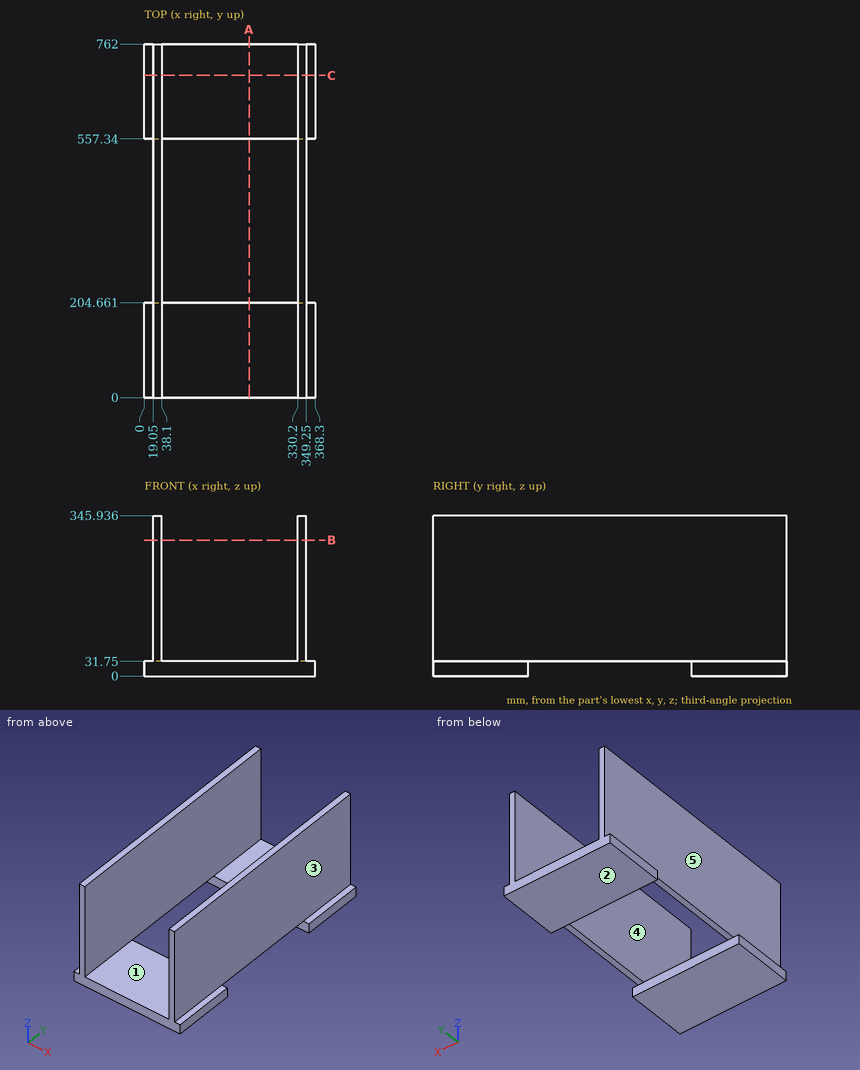
The drawing under review shows one solid part. Ordinate dimensions are in mm from its lowest x, y, z. A direction names the side the tool comes from. Coordinates: 2 decimals unless noted, no trailing zeros. Order: outer loops, then holes, each group sorted by start corner. A loop starts at its lowest first (then second) coordinate and runs counter-clockwise, first axis right, second up. Notation, with made-up numbers: (-21, 60) -> (23, 60) arc R16 ccw to (23, 88) -> close; hole circle Ø2 at (-19.5, 63.5). An arc over 180 degrees is marked (long way). One line per item, written item: value.
1) We need section B-B, the plane z = 293. Give the boundary of the cut face in (x, y), then the cut area to 3 significant figures.
Output values:
outline: (19.05, 0) -> (38.1, 0) -> (38.1, 762) -> (19.05, 762) -> close; (330.2, 0) -> (349.25, 0) -> (349.25, 762) -> (330.2, 762) -> close
area: 29,000 mm2
2) To check wall thickness, follow probe 1 along X at (y, z) = (91, 131); probe 2 along Z at (x, y) = (287.5, 100); probe 3 along Y at (x, z) = (144.5, 22.5). State the ranges of each line that lie inside material, in increasing order. Write a range as [from, to].
Output values:
probe 1: x = [19.05, 38.1], [330.2, 349.25]
probe 2: z = [0, 31.75]
probe 3: y = [0, 204.66], [557.34, 762]
3) Machinability: for the marked faces 1 and 2, which of the approach directions +Z, -Z, +X, -X, +Y, -Y give a long, thin tool a straight path to every point of the face, cutting with its end or side? Answer none if there is none.
Output values:
face 1: +Z, +Y, -Y
face 2: -Z, +X, -X, +Y, -Y
4) Draft analysis for pull direction X (two halves, no side actions). For the marked faces 3, 4 and 5, state which applies: +X half, -X half, draft (parallel to the pull), parting line (faces both ways), or undercut.
Output values:
face 3: +X half
face 4: undercut
face 5: -X half
5) We need section A-A, the plane x = 226. Give the boundary of the cut face in (y, z).
Output values:
outline: (0, 0) -> (204.66, 0) -> (204.66, 31.75) -> (0, 31.75) -> close; (557.34, 0) -> (762, 0) -> (762, 31.75) -> (557.34, 31.75) -> close
6) We need section C-C, the plane y = 694.5. Give the boundary of the cut face in (x, z), then the cut area to 3 significant figures.
Output values:
outline: (0, 0) -> (368.3, 0) -> (368.3, 31.75) -> (349.25, 31.75) -> (349.25, 345.94) -> (330.2, 345.94) -> (330.2, 31.75) -> (38.1, 31.75) -> (38.1, 345.94) -> (19.05, 345.94) -> (19.05, 31.75) -> (0, 31.75) -> close
area: 23,700 mm2
7) Clearance check with flat-ended pins moving along their axes: P1, Ø5.5, axis at x = 361, y = 106.5, coming from the +Z side; P2, Ø5.5, axis at x = 29, y = 321, coming from the -Z side; P3, Ø15, axis at x = 12.5, y = 125, coming from the +Z side; P4, Ø3, axis at y = 521, z = 63.5, coming from the -X side. State where each tip first meets the part, or that it passes through.
Output values:
P1: stops at z = 31.75
P2: stops at z = 31.75
P3: stops at z = 345.94
P4: stops at x = 19.05
